```python
from build123d import *

# Parameters (mm, degrees)
RECTANGULAR_TUBE_CONFIGURED_50_X_30_X_DEPTH = 34.4
M5_CLEARANCE_HOLE1_D                        = 5.5


with BuildPart() as part:
    # Sketch13 → Rectangular tube - configured 50 X 30 X 2.6(1) (new body)
    with BuildSketch(Plane(origin=(0, 0, 0), x_dir=(1, 0, 0), z_dir=(0, 1, 0))):
        with BuildLine():
            Line((-9.8, -25), (9.8, -25))
            ThreePointArc((9.8, -25), (13.476955262, -23.476955262), (15, -19.8))
            Line((15, -19.8), (15, 19.8))
            ThreePointArc((15, 19.8), (13.476955262, 23.476955262), (9.8, 25))
            Line((9.8, 25), (-9.8, 25))
            ThreePointArc((-9.8, 25), (-13.476955262, 23.476955262), (-15, 19.8))
            Line((-15, 19.8), (-15, -19.8))
            ThreePointArc((-15, -19.8), (-13.476955262, -23.476955262), (-9.8, -25))
        make_face()
        with BuildLine():
            Line((-9.8, -22.4), (9.8, -22.4))
            ThreePointArc((9.8, -22.4), (11.638477631, -21.638477631), (12.4, -19.8))
            Line((12.4, -19.8), (12.4, 19.8))
            ThreePointArc((12.4, 19.8), (11.638477631, 21.638477631), (9.8, 22.4))
            Line((9.8, 22.4), (-9.8, 22.4))
            ThreePointArc((-9.8, 22.4), (-11.638477631, 21.638477631), (-12.4, 19.8))
            Line((-12.4, 19.8), (-12.4, -19.8))
            ThreePointArc((-12.4, -19.8), (-11.638477631, -21.638477631), (-9.8, -22.4))
        make_face(mode=Mode.SUBTRACT)
    extrude(amount=RECTANGULAR_TUBE_CONFIGURED_50_X_30_X_DEPTH)

    # M5 Clearance Hole1 (through all)
    with Locations(Plane(origin=(0, 26.435, 25), x_dir=(1, 0, 0), z_dir=(0, 0, 1))):
        with Locations((0, 0), (0, -18.47)):
            Hole(M5_CLEARANCE_HOLE1_D / 2)


solid = part.part
```
Check sheet for the modelled part. Datum: model origin and axes. Units: mm. A direction names the side the tool comes from. Give positions to 0.01 mm unless a question says otherwise; leave off trailing zeros. Write each loop counter-clockwise with the first axis right and the second up, starting at its lowest first coordinate (ties: lowest second). Pieces come first, ordered by that corner, then holes. Notation, with made-up numbers: (53, 53) -> (79, 53) arc R15 ccw to (79, 75) -> close; hole circle Ø7 at (13, 7). An arc over 180 degrees is marked (long way). Use CSV: the item, a comma, the result in double quotes. Start each with the question number.
Q1. Tool access check on faces 5 (the cylindrical face through (-11.659, 16.959, 21.618)), 6 (the flat face through (0, 17, 25)). Record the directions out of +Z, -Z, +X, -X, +Y, -Y that give a thin tool (end or side, any length) a straight path to the whole face; none if there is none.
Q2. Cross-section at A-A on z = 16. Enter the section's corners in (x, y), and give its area (3 significant figures).
Q3. Release check for a two-part mould opening along X. For faces 1 (the flat face through (-12.4, 17, 0)), 2 (the flat face through (0, 17, -22.4)), 3 (the flat face through (-13, 0, 0)), 4 (the cylindrical face through (13.436, 16.959, 23.517)) record: +X half, -X half, draft (parallel to the pull), parting line (faces both ways), or undercut.
Q4. Depth check by flat-ended pin: P1, Ø10, axis at x = 0.5, y = 25, coming from the +Z side. Enter the tip coordinate at first touch or a pass-through.
Q5. Cross-section at C-C on y = 27.5. Enter the section's corners in (x, z), and give its area (3 significant figures).
Q6. Cross-section at B-B on x = 0. Enter the section's corners in (y, z) (3 decimals), and give its area (3 significant figures).
Q7. Cross-section at D-D on x = -10.75. Enter the section's corners in (y, z).
Q8. Scan lines: line 1 along Y through (x, z) = (0, 24.45) (3 decimals); line 2 along X through (y, z) = (27, -9.5); line 3 along Z through (x, y) = (2.75, 31). Record each from-to range of solid material in increasing order.
Working result:
1,face 5,"+Y, -Y"
1,face 6,"+Z, +X, -X, +Y, -Y"
2,outline,"(-15, 0) -> (-12.4, 0) -> (-12.4, 34.4) -> (-15, 34.4) -> close; (12.4, 0) -> (15, 0) -> (15, 34.4) -> (12.4, 34.4) -> close"
2,area,"179 mm^2"
3,face 1,"undercut"
3,face 2,"undercut"
3,face 3,"draft"
3,face 4,"+X half"
4,P1,"stops at z = 25"
5,outline,"(-15, -19.8) arc R5.2 ccw to (-9.8, -25) -> (-2.54, -25) -> (-2.54, -22.4) -> (-9.8, -22.4) arc R2.6 cw to (-12.4, -19.8) -> (-12.4, 19.8) arc R2.6 cw to (-9.8, 22.4) -> (-2.54, 22.4) -> (-2.54, 25) -> (-9.8, 25) arc R5.2 ccw to (-15, 19.8) -> close; (2.54, -25) -> (9.8, -25) arc R5.2 ccw to (15, -19.8) -> (15, 19.8) arc R5.2 ccw to (9.8, 25) -> (2.54, 25) -> (2.54, 22.4) -> (9.8, 22.4) arc R2.6 cw to (12.4, 19.8) -> (12.4, -19.8) arc R2.6 cw to (9.8, -22.4) -> (2.54, -22.4) -> close"
5,area,"345 mm^2"
6,outline,"(0, -25) -> (5.215, -25) -> (5.215, -22.4) -> (0, -22.4) -> close; (0, 22.4) -> (5.215, 22.4) -> (5.215, 25) -> (0, 25) -> close; (10.715, -25) -> (23.685, -25) -> (23.685, -22.4) -> (10.715, -22.4) -> close; (10.715, 22.4) -> (23.685, 22.4) -> (23.685, 25) -> (10.715, 25) -> close; (29.185, -25) -> (34.4, -25) -> (34.4, -22.4) -> (29.185, -22.4) -> close; (29.185, 22.4) -> (34.4, 22.4) -> (34.4, 25) -> (29.185, 25) -> close"
6,area,"122 mm^2"
7,outline,"(0, -24.91) -> (34.4, -24.91) -> (34.4, -22.22) -> (0, -22.22) -> close; (0, 22.22) -> (34.4, 22.22) -> (34.4, 24.91) -> (0, 24.91) -> close"
8,line 1,"y = 0 to 5.215, 10.715 to 23.685, 29.185 to 34.4"
8,line 2,"x = -15 to -12.4, 12.4 to 15"
8,line 3,"z = -25 to -22.4, 22.4 to 25"
